Design review of the part built by this model. Coordinates are the model's own, in mm. A direction names the side the tool comes from. Give positions to 0.01 mm unless a question says otherwise; leave off trailing zeros. Loops run counter-clockwise (first coordinate to the right, second up) from the corner with the lowest first, then second, coordinate; pieces in that order, holes last. Notation, with made-up numbers: M 30,-15 L 74,-15 A20 ccw 74,-1 Z; hole C -20,26.25 d11. An arc over 180 degrees is marked long. Use one line per item in the form item = value. Start each with the question number.
from build123d import *

# Parameters (mm, degrees)
SKETCH1_W                      = 25.019
SKETCH1_H                      = 6.6802
BOSS_EXTRUDE1_DEPTH            = 7.62
SKETCH2_W                      = 19.9898
SKETCH2_H                      = 1.651
CUT_EXTRUDE1_DEPTH             = 1.778
SKETCH5_W                      = 19.9898
SKETCH5_H                      = 2.5146
BOSS_EXTRUDE2_DEPTH            = 6.731
CUT_EXTRUDE2_REACH             = 18.974
SKETCH7_W                      = 8.1026
SKETCH7_H                      = 6.731
CUT_EXTRUDE2_DIRECTION_2_DEPTH = 17.973785465
CUT_EXTRUDE5_REACH             = 18.974
SKETCH8_R                      = 1.5748
SKETCH8_R_2                    = 0.4826
SKETCH8_R_3                    = 0.508
SKETCH9_W                      = 25.019
SKETCH9_H                      = 5.08
BOSS_EXTRUDE3_DEPTH            = 12.7


with BuildPart() as part:
    # Sketch1 → Boss-Extrude1 (new body)
    with BuildSketch(Plane(origin=(0, 0, 0), x_dir=(1, 0, 0), z_dir=(0, 1, 0))):
        with Locations((1.107398361, 2.278921311)):
            Rectangle(SKETCH1_W, SKETCH1_H)
    extrude(amount=BOSS_EXTRUDE1_DEPTH)

    # Sketch2 → Cut-Extrude1 (cut)
    with BuildSketch(Plane.XZ):
        with Locations((1.107398361, -2.278921311)):
            Rectangle(SKETCH2_W, SKETCH2_H)
    extrude(amount=-CUT_EXTRUDE1_DEPTH, mode=Mode.SUBTRACT)

    # Sketch5 → Boss-Extrude2 (add)
    with BuildSketch(Plane.XZ):
        with Locations((1.107398361, -0.196121311)):
            Rectangle(SKETCH5_W, SKETCH5_H)
    extrude(amount=BOSS_EXTRUDE2_DEPTH)

    # Sketch7 → Cut-Extrude2 (cut, up to next)
    with BuildSketch(Plane.XY.offset(1.061178689), mode=Mode.PRIVATE) as cut_extrude2_sk1:
        with Locations((3.799798361, -3.3655)):
            Rectangle(SKETCH7_W, SKETCH7_H)
    cut_extrude2_tool1 = extrude(cut_extrude2_sk1.sketch, amount=-CUT_EXTRUDE2_REACH, mode=Mode.PRIVATE) & part.part
    add(cut_extrude2_tool1.solids().sort_by_distance((3.799798, -3.3655, 1.061179))[0], mode=Mode.SUBTRACT)

    # Sketch7 → Cut-Extrude2 direction 2 (cut)
    with BuildSketch(Plane.XY.offset(1.061178689)):
        with Locations((3.799798361, -3.3655)):
            Rectangle(SKETCH7_W, SKETCH7_H)
    extrude(amount=CUT_EXTRUDE2_DIRECTION_2_DEPTH, mode=Mode.SUBTRACT)

    # Sketch8 → Cut-Extrude5 (cut, up to next)
    with BuildSketch(Plane.XY.offset(1.061178689), mode=Mode.PRIVATE) as cut_extrude5_sk1:
        with Locations((-6.347501639, -0.762)):
            Circle(SKETCH8_R)
    cut_extrude5_tool1 = extrude(cut_extrude5_sk1.sketch, amount=-CUT_EXTRUDE5_REACH, mode=Mode.PRIVATE) & part.part
    # Sketch8 → Cut-Extrude5 (cut, up to next)
    with BuildSketch(Plane.XY.offset(1.061178689), mode=Mode.PRIVATE) as cut_extrude5_sk2:
        with Locations((9.832298361, -2.413)):
            Circle(SKETCH8_R_2)
    cut_extrude5_tool2 = extrude(cut_extrude5_sk2.sketch, amount=-CUT_EXTRUDE5_REACH, mode=Mode.PRIVATE) & part.part
    # Sketch8 → Cut-Extrude5 (cut, up to next)
    with BuildSketch(Plane.XY.offset(1.061178689), mode=Mode.PRIVATE) as cut_extrude5_sk3:
        with Locations((9.832298361, -4.953)):
            Circle(SKETCH8_R_3)
    cut_extrude5_tool3 = extrude(cut_extrude5_sk3.sketch, amount=-CUT_EXTRUDE5_REACH, mode=Mode.PRIVATE) & part.part
    add(cut_extrude5_tool1.solids().sort_by_distance((-6.347502, -0.762, 1.061179))[0], mode=Mode.SUBTRACT)
    add(cut_extrude5_tool2.solids().sort_by_distance((9.832298, -2.413, 1.061179))[0], mode=Mode.SUBTRACT)
    add(cut_extrude5_tool3.solids().sort_by_distance((9.832298, -4.953, 1.061179))[0], mode=Mode.SUBTRACT)

    # Sketch9 → Boss-Extrude3 (add)
    with BuildSketch(Plane.XY.offset(1.061178689)):
        with Locations((1.107398361, 5.08)):
            Rectangle(SKETCH9_W, SKETCH9_H)
    extrude(amount=BOSS_EXTRUDE3_DEPTH)


solid = part.part
Q1. The part is to be moulded in two halves that separate along Y. For faces 5 (the cylindrical face through (-4.893, -1.365, -0.179)), 6 (the flat face through (-5, -6.731, 0)), 7 (the flat face through (7.851, -3, 0)), say which applies: pulls with the +Y half, pulls with the -Y half, needs draft (parallel to the pull), parting line crosses it, or undercut.
Q2. Wall thickness on probe 1 along Z at (x, y) = (-2.75, 1); probe 2 along Z at (x, y) = (10.5, -2); probe 3 along Y at (x, z) = (-8.5, -3.5): over which ranges is each line inside the solid? List them lowest first.
Q3. For faces 1 (the flat face through (1, 2.54, 7)), 2 (the flat face through (1, 1.778, -2)), 3 (the flat face through (11.102, -3, 0)), 4 (the flat face through (-8.888, -3, 0)), list the 3-axis set-ups (+Z, -Z, +X, -X, +Y, -Y) from which the entire face can be reached by the end or side of a thin tool; tool diameter is ignored.
Q4. Take a section at B-B on y = -1.25. Give the boundary of the cut face in (x, z), plus the area to 3 significant figures.
Q5. Take a section at A-A on z = -2.75. Give the boundary of the cut face in (x, y).
Q6. Clearance check with flat-ended pins moving along their axes: pin 1 Ø2 at (y, z) = (-3, -1) entering from +X; pin 2 Ø2 at (x, z) = (3, -1) entering from -Y; pin 3 Ø2.5 at (x, y) = (-6.35, -0.76) entering from +Z. State where each tip first meets the part, or that it passes through.
Q7. Take a section at C-C on x = -7. Give the boundary of the cut face in (y, z), plus the area to 3 significant figures.
Q8. Take a section at D-D on x = -2.5. Give the boundary of the cut face in (y, z).
Response values:
q1.face_5 = undercut
q1.face_6 = pulls with the -Y half
q1.face_7 = needs draft
q2.probe_1 = -5.62 to -3.1, -1.45 to 1.06
q2.probe_2 = -1.45 to 1.06
q2.probe_3 = 0 to 7.62
q3.face_1 = +Z, +X, -X, -Y
q3.face_2 = -Y
q3.face_3 = +Z, -Z, +X, -Y
q3.face_4 = +Z, -Z, -X, -Y
q4.outline = M -8.89,-1.45 L -7.84,-1.45 L -7.84,1.06 L -8.89,1.06 Z; M -4.85,-1.45 L -0.25,-1.45 L -0.25,1.06 L -4.85,1.06 Z; M 7.85,-1.45 L 11.1,-1.45 L 11.1,1.06 L 7.85,1.06 Z
q4.area = 22.4 mm^2
q5.outline = M -11.4,0 L -8.89,0 L -8.89,1.78 L 11.1,1.78 L 11.1,0 L 13.62,0 L 13.62,7.62 L -11.4,7.62 Z
q6.pin_1 = 11.1
q6.pin_2 = 0
q6.pin_3 = -3.1
q7.outline = M -6.73,-1.45 L -2.2,-1.45 L -2.2,1.06 L -6.73,1.06 Z; M 0,-5.62 L 7.62,-5.62 L 7.62,13.76 L 2.54,13.76 L 2.54,1.06 L 0.67,1.06 L 0.67,-1.45 L 1.78,-1.45 L 1.78,-3.1 L 0,-3.1 Z
q7.area = 122 mm^2
q8.outline = M -6.73,-1.45 L 1.78,-1.45 L 1.78,-3.1 L 0,-3.1 L 0,-5.62 L 7.62,-5.62 L 7.62,13.76 L 2.54,13.76 L 2.54,1.06 L -6.73,1.06 Z
